Work out the finished part from the listing and answer in its coordinate system (mm). A direction names the side the tool comes from. Give positions to 0.01 mm unless a question says otherwise; leave off trailing zeros. Write each loop counter-clockwise with the first axis right and the second up, starting at its lowest first coordinate (ties: lowest second). Pieces come first, ordered by that corner, then holes. Notation, with made-up numbers: (53.5, -1) -> (79.5, -1) arc R12 ccw to (79.5, 18) -> close; hole circle Ø2 at (47.5, -27). An arc over 180 degrees is marked (long way). Use a Markdown table: item, result. Add a question column.
Q1. Section B-B, the plane x = 2.5 is taken. Give the vertices of the cut face in (y, z), plus the area to 3 significant figures.
Q2. Consider line 1 (Y direction, x = 4, z = 8); line 2 (X direction, y = 2, z = 12.5); line 3 (X direction, y = 4.5, z = 5). Determine where each line is inside the solid, lowest interval first.
Q3. For faces 5 (the face through (0, 32, 22)), 6 (the face through (15, -12.8, 12.7)), 7 (the face through (11.99, 10.15, 35.14)), determine the directions among +Z, -Z, +X, -X, +Y, -Y from which every point of the face is accessible in a straight line to the end or side of a thin tool.
Q4. Section A-A, the plane y = -1.5 is taken. Give the vertices of the cut face in (x, z), plus the area to 3 significant figures.
Q5. Section C-C, the plane z = 42 is taken. Give the vertices of the cut face in (x, y), plus the area to 3 significant figures.
Q6. Each of these flat-tipped pins is pushed along its axis until it touches: pin 1 Ø8 at (x, z) = (-22, 20) entering from -Y; pin 2 Ø1 at (x, z) = (-10.5, 14) entering from -Y; pin 3 Ø1.5 at (y, z) = (19, 39) entering from -X. Where does it stop, or does it pass through?
Q7. Section D-D, the plane z = 22 is taken. Give the vertices of the cut face in (x, y), plus the area to 3 significant figures.
Q8. For a pull along X with two mould halves and no side action, classify faces 1 (the face through (-12.15, -9.99, 35.14)), 2 (the face through (34, 0, 22)), 3 (the face through (14.8, 13, 12.7)), 4 (the face through (-26.871, -24.482, 22.815)) as pulls with the +X half, pulls with the -X half, needs draft (parallel to the pull), parting line crosses it, or undercut.
from build123d import *

# Parameters (mm, degrees)
F0_W     = 68
F0_H     = 64
F0_W_2   = 38
F0_H_2   = 34
F1_DEPTH = 25
F2_W     = 68
F2_H     = 64
F2_W_2   = 38
F2_H_2   = 34
F2_W_3   = 29.9999998808
F2_H_3   = 25.9999998808
F3_DEPTH = 20
F4_R     = 10
F5_R     = 14
F6_R     = 25


with BuildPart() as f1:
    # F0 (on Top) → F1 (new body)
    with BuildSketch(Plane.XY):
        Rectangle(F0_W, F0_H)
        Rectangle(F0_W_2, F0_H_2, mode=Mode.SUBTRACT)
    extrude(amount=F1_DEPTH)

    # F2 (on face) → F3 (join)
    with BuildSketch(Plane.XY.offset(25)):
        Rectangle(F2_W, F2_H)
        Rectangle(F2_W_2, F2_H_2, mode=Mode.SUBTRACT)
        Rectangle(F2_W_2, F2_H_2)
        Rectangle(F2_W_3, F2_H_3, mode=Mode.SUBTRACT)
    extrude(amount=F3_DEPTH)

    # F4
    f4_edges = [f1.edges().sort_by_distance(p)[0] for p in [
        (-15, 13, 35),
        (-15, -13, 35),
        (15, -13, 35),
        (15, 13, 35),
    ]]
    fillet(f4_edges, radius=F4_R)

    # F5
    f5_edges = [f1.edges().sort_by_distance(p)[0] for p in [
        (19, -17, 12.5),
        (19, 17, 12.5),
        (-19, 17, 12.5),
        (-19, -17, 12.5),
    ]]
    fillet(f5_edges, radius=F5_R)

    # F6
    f6_edges = [f1.edges().sort_by_distance(p)[0] for p in [
        (34, 32, 22.5),
        (-34, 32, 22.5),
        (34, -32, 22.5),
        (-34, -32, 22.5),
    ]]
    fillet(f6_edges, radius=F6_R)


solid = f1.part
Result set:
| question | item | result |
|---|---|---|
| 1 | outline | (-32, 0) -> (-17, 0) -> (-17, 25) -> (-13, 25) -> (-13, 45) -> (-32, 45) -> close; (13, 25) -> (17, 25) -> (17, 0) -> (32, 0) -> (32, 45) -> (13, 45) -> close |
| 1 | area | 1,510 mm2 |
| 2 | line 1 | y = -32 to -17, 17 to 32 |
| 2 | line 2 | x = -34 to -19, 19 to 34 |
| 2 | line 3 | x = -34 to -18.92, 18.92 to 34 |
| 3 | face 5 | +Z, -Z, +X, -X, +Y |
| 3 | face 6 | -Z |
| 3 | face 7 | +Z, -Z |
| 4 | outline | (-34, 0) -> (-19, 0) -> (-19, 25) -> (-15, 25) -> (-15, 45) -> (-34, 45) -> close; (15, 25) -> (19, 25) -> (19, 0) -> (34, 0) -> (34, 45) -> (15, 45) -> close |
| 4 | area | 1,510 mm2 |
| 5 | outline | (-34, -7) arc R25 ccw to (-9, -32) -> (9, -32) arc R25 ccw to (34, -7) -> (34, 7) arc R25 ccw to (9, 32) -> (-9, 32) arc R25 ccw to (-34, 7) -> close; hole (-15, -3) arc R10 ccw to (-5, -13) -> (5, -13) arc R10 ccw to (15, -3) -> (15, 3) arc R10 ccw to (5, 13) -> (-5, 13) arc R10 ccw to (-15, 3) -> close |
| 5 | area | 3,120 mm2 |
| 6 | pin 1 | stops at y = -30.32 |
| 6 | pin 2 | stops at y = -31.98 |
| 6 | pin 3 | stops at x = -31.33 |
| 7 | outline | (-34, -7) arc R25 ccw to (-9, -32) -> (9, -32) arc R25 ccw to (34, -7) -> (34, 7) arc R25 ccw to (9, 32) -> (-9, 32) arc R25 ccw to (-34, 7) -> close; hole (-19, -3) arc R14 ccw to (-5, -17) -> (5, -17) arc R14 ccw to (19, -3) -> (19, 3) arc R14 ccw to (5, 17) -> (-5, 17) arc R14 ccw to (-19, 3) -> close |
| 7 | area | 2,690 mm2 |
| 8 | face 1 | undercut |
| 8 | face 2 | pulls with the +X half |
| 8 | face 3 | undercut |
| 8 | face 4 | pulls with the -X half |
